Can you work these out from the model? Positions are in its coordinate system, mm. A direction names the side the tool comes from. Coordinates: 2 decimals unless noted, no trailing zeros. Order: outer loops, then holes, each group sorted by start corner. A loop starts at its lowest first (then second) coordinate and runs counter-clockwise, first axis right, second up.
```python
from build123d import *

# Parameters (mm, degrees)
EXTRUDE_1_DEPTH = 60
SKETCH_2_R      = 7.5
EXTRUDE_2_DEPTH = 50


with BuildPart() as part:
    # 草圖1 → 填料-伸長1 (new body)
    with BuildSketch(Plane.XY):
        Polygon((0, 0), (70, 0), (70, 24), (32, 60), (0, 60), align=None)
    extrude(amount=EXTRUDE_1_DEPTH)

    # 草圖2 → 填料-伸長2 (add)
    with BuildSketch(Plane(origin=(45.091970803, 47.597080292, 0), x_dir=(0.7259526839058265, -0.6877446479107832, 0), z_dir=(0.6877446479107832, 0.7259526839058265, 0))):
        with Locations(Location((9.310816324, -30, 0), (0, 0, 180))):
            Circle(SKETCH_2_R)
    extrude(amount=EXTRUDE_2_DEPTH)


solid = part.part
```
1. I'm going to push flat-ended pins straight in: pin 1 (3 mm diameter, centred on y = 40.5, z = 46, fed in from +X); pin 2 (7 mm diameter, centred on y = 11.5, z = 19, fed in from +X); pin 3 (2 mm diameter, centred on x = 44, z = 17, fed in from +Y). Where does each tip first touch, or does it pass through?
Completed:
pin 1: stops at x = 54.17
pin 2: stops at x = 70
pin 3: stops at y = 49.58
2. Thinking about a two-plate mould opening in Y: for faces 1 (the flat face through (16, 60, 30)), 2 (the flat face through (0, 30, 30)), 3 (the cylindrical face through (69.984, 57.97, 22.678)), which applies, pulls with the +Y half, pulls with the -Y half, needs draft (parallel to the pull), parting line crosses it, or undercut?
Completed:
face 1: pulls with the +Y half
face 2: needs draft
face 3: undercut
3. Imagine slicing it at B-B on z = 16.5. Please give me the cut outline in (x, y), then the cut area to 3 significant figures.
Completed:
outline: (0, 0) - (70, 0) - (70, 24) - (32, 60) - (0, 60) - close
area: 3,520 mm2
4. Please list where these lines run through material, in increasing order: probe 1 along X at (y, z) = (22, 52); probe 2 along Y at (x, z) = (11.5, 45); probe 3 along Y at (x, z) = (62.5, 27).
Completed:
probe 1: x = 0 to 70
probe 2: y = 0 to 60
probe 3: y = 0 to 31.11, 42.44 to 62.43
5. Imagine slicing it at A-A on y = 8. Please give me the cut outline in (x, z).
Completed:
outline: (0, 0) - (70, 0) - (70, 60) - (0, 60) - close
6. On a 3-axis mill with a long thin cutter (end or side, diameter ignored), from which of +Z, -Z, +X, -X, +Y, -Y can I reach the whole of each face in a straight line? I mean faces 4 (the flat face through (55.488, 37.748, 36.247)), 5 (the flat face through (35, 0, 30)), 6 (the flat face through (70, 12, 30)). Say none if no direction works.
Completed:
face 4: none
face 5: +Z, -Z, +X, -X, -Y
face 6: +Z, -Z, +X, -Y
7. Imagine slicing it at C-C on x = 14. Please give me the cut outline in (y, z), then the cut area to 3 significant figures.
Completed:
outline: (0, 0) - (60, 0) - (60, 60) - (0, 60) - close
area: 3,600 mm2
